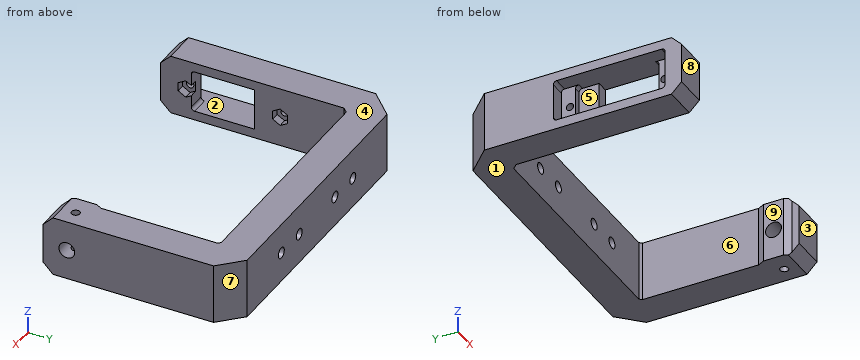
```python
from build123d import *

# Parameters (mm, degrees)
BOSS_EXTRUDE1_DEPTH             = 9
SKETCH2_R                       = 0.5
CUT_EXTRUDE1_DEPTH              = 67.414213562
SKETCH9_R                       = 2.38125
PIN_HOLE_DEPTH                  = 93.121320344
SKETCH20_R                      = 1.21925
SPRING_PIN_DEPTH                = 10
SPRING_PIN_DEPTH_BACK           = 10
SKETCH32_W                      = 12.5
SKETCH32_H                      = 33.5
CUT_EXTRUDE11_DEPTH             = 4.5
CUT_EXTRUDE12_REACH             = 89.621
SKETCH33_W                      = 12.5
SKETCH33_H                      = 25
CUT_EXTRUDE13_REACH             = 89.621
SKETCH34_R                      = 1.1
FILLET1_R                       = 1
TAP_DRILL_FOR_M4X0_7_TAP1_D     = 3.3
TAP_DRILL_FOR_M4X0_7_TAP1_DEPTH = 66.414213562
SKETCH41_W                      = 12.5
SKETCH41_H                      = 6
BOSS_EXTRUDE4_DEPTH             = 3.5
CUT_EXTRUDE14_DEPTH             = 2.5
BOSS_EXTRUDE6_DEPTH             = 9
CHAMFER1_SIZE                   = 3
CUT_EXTRUDE15_REACH             = 84.121
SKETCH45_R                      = 2.38125


with BuildPart() as part:
    # Sketch1 → Boss-Extrude1 (new body, symmetric)
    with BuildSketch(Plane.XY):
        Polygon((-35, 0), (35, 0), (35.707106781, -0.707106781), (35.707106781, -47.707106781), (45.707106781, -47.707106781), (45.707106781, 3.435028843), (39.142135624, 10), (-39.142135624, 10), (-46.414213562, 2.727922061), (-46.414213562, -56.414213562), (-36.414213562, -56.414213562), (-36.414213562, -1.414213562), align=None)
    extrude(amount=BOSS_EXTRUDE1_DEPTH, both=True)

    # Sketch2 → Cut-Extrude1 (cut, through all)
    with BuildSketch(Plane(origin=(0, 10, 0), x_dir=(1, 0, 0), z_dir=(0, 1, 0))):
        with Locations((-10, 0)):
            Circle(SKETCH2_R)
        with Locations((10, 0)):
            Circle(SKETCH2_R)
        with Locations((-20, 0)):
            Circle(SKETCH2_R)
        with Locations((20, 0)):
            Circle(SKETCH2_R)
    extrude(amount=-CUT_EXTRUDE1_DEPTH, mode=Mode.SUBTRACT)

    # Sketch9 → Pin Hole (cut, through all)
    with BuildSketch(Plane(origin=(45.707106781, 0, 0), x_dir=(0, 0, -1), z_dir=(1, 0, 0))):
        with Locations((0, -40.564971157)):
            Circle(SKETCH9_R)
    extrude(amount=-PIN_HOLE_DEPTH, mode=Mode.SUBTRACT)

    # Sketch20 → spring pin (cut, two sides)
    with BuildSketch(Plane.XY) as spring_pin_sk:
        with Locations((40.707106781, -40.564971157)):
            Circle(SKETCH20_R)
    extrude(amount=SPRING_PIN_DEPTH, mode=Mode.SUBTRACT)
    extrude(spring_pin_sk.sketch, amount=-SPRING_PIN_DEPTH_BACK, mode=Mode.SUBTRACT)

    # Sketch32 → Cut-Extrude11 (cut)
    with BuildSketch(Plane.ZY.offset(46.414213562)):
        with Locations((0, -34.734971157)):
            Rectangle(SKETCH32_W, SKETCH32_H)
    extrude(amount=-CUT_EXTRUDE11_DEPTH, mode=Mode.SUBTRACT)

    # Sketch33 → Cut-Extrude12 (cut, up to next)
    with BuildSketch(Plane.ZY.offset(41.914213562), mode=Mode.PRIVATE) as cut_extrude12_sk1:
        with Locations((0, -34.734971157)):
            Rectangle(SKETCH33_W, SKETCH33_H)
    cut_extrude12_tool1 = extrude(cut_extrude12_sk1.sketch, amount=-CUT_EXTRUDE12_REACH, mode=Mode.PRIVATE) & part.part
    add(cut_extrude12_tool1.solids().sort_by_distance((-41.914214, -34.734971, 0))[0], mode=Mode.SUBTRACT)

    # Sketch34 → Cut-Extrude13 (cut, up to next)
    with BuildSketch(Plane.ZY.offset(41.914213562), mode=Mode.PRIVATE) as cut_extrude13_sk1:
        with Locations((0, -20.574371157)):
            Circle(SKETCH34_R)
    cut_extrude13_tool1 = extrude(cut_extrude13_sk1.sketch, amount=-CUT_EXTRUDE13_REACH, mode=Mode.PRIVATE) & part.part
    add(cut_extrude13_tool1.solids().sort_by_distance((-41.914214, -20.574371, 0))[0], mode=Mode.SUBTRACT)
    # Sketch34 → Cut-Extrude13 (cut, up to next)
    with BuildSketch(Plane.ZY.offset(41.914213562), mode=Mode.PRIVATE) as cut_extrude13_sk2:
        with Locations((0, -48.895371157)):
            Circle(SKETCH34_R)
    cut_extrude13_tool2 = extrude(cut_extrude13_sk2.sketch, amount=-CUT_EXTRUDE13_REACH, mode=Mode.PRIVATE) & part.part
    add(cut_extrude13_tool2.solids().sort_by_distance((-41.914214, -48.895371, 0))[0], mode=Mode.SUBTRACT)

    # Fillet1
    fillet1_edges = [part.edges().sort_by_distance(p)[0] for p in [
        (-44.164213562, -17.984971157, 6.25),
        (-44.164213562, -51.484971157, 6.25),
        (-44.164213562, -51.484971157, -6.25),
        (-44.164213562, -17.984971157, -6.25),
        (-39.164213562, -22.234971157, -6.25),
        (-39.164213562, -47.234971157, -6.25),
        (-39.164213562, -47.234971157, 6.25),
        (-39.164213562, -22.234971157, 6.25),
    ]]
    fillet(fillet1_edges, radius=FILLET1_R)

    # Tap Drill for M4x0.7 Tap1
    with Locations(Plane(origin=(0, 10, 0), x_dir=(1, 0, 0), z_dir=(0, 1, 0))):
        with Locations((-20, 0), (20, 0), (-10, 0), (10, 0)):
            Hole(TAP_DRILL_FOR_M4X0_7_TAP1_D / 2, depth=TAP_DRILL_FOR_M4X0_7_TAP1_DEPTH)

    # Sketch41 → Boss-Extrude4 (add)
    with BuildSketch(Plane(origin=(-36.414213562, 0, 0), x_dir=(0, 0, -1), z_dir=(1, 0, 0))):
        with Locations((0, -25.234971157)):
            Rectangle(SKETCH41_W, SKETCH41_H)
    extrude(amount=-BOSS_EXTRUDE4_DEPTH)

    # Sketch43 → Cut-Extrude14 (cut)
    with BuildSketch(Plane(origin=(-36.414213562, 0, 0), x_dir=(0, 0, -1), z_dir=(1, 0, 0))):
        Polygon((-1.299038106, -22.824371157), (1.299038106, -22.824371157), (2.598076211, -20.574371157), (1.299038106, -18.324371157), (-1.299038106, -18.324371157), (-2.598076211, -20.574371157), align=None)
        Polygon((-1.299038106, -46.645371157), (-2.598076211, -48.895371157), (-1.299038106, -51.145371157), (1.299038106, -51.145371157), (2.598076211, -48.895371157), (1.299038106, -46.645371157), align=None)
    extrude(amount=-CUT_EXTRUDE14_DEPTH, mode=Mode.SUBTRACT)

    # Sketch44 → Boss-Extrude6 (add, symmetric)
    with BuildSketch(Plane.XY):
        Polygon((34.707106781, -37.564971157), (34.707106781, -40.564971157), (35.707106781, -40.564971157), (35.707106781, -35.564971157), align=None)
        Polygon((34.707106781, -40.564971157), (34.707106781, -43.564971157), (35.707106781, -45.564971157), (35.707106781, -40.564971157), align=None)
    extrude(amount=BOSS_EXTRUDE6_DEPTH, both=True)

    # Chamfer1
    chamfer1_edges = [part.edges().sort_by_distance(p)[0] for p in [
        (40.707106781, -47.707106781, -9),
        (40.707106781, -47.707106781, 9),
        (-41.414213562, -56.414213562, -9),
        (-41.414213562, -56.414213562, 9),
    ]]
    chamfer(chamfer1_edges, length=CHAMFER1_SIZE)

    # Sketch45 → Cut-Extrude15 (cut, up to next)
    with BuildSketch(Plane(origin=(35.707106781, 0, 0), x_dir=(0, 0, -1), z_dir=(1, 0, 0)), mode=Mode.PRIVATE) as cut_extrude15_sk1:
        with Locations((0, -40.564971157)):
            Circle(SKETCH45_R)
    cut_extrude15_tool1 = extrude(cut_extrude15_sk1.sketch, amount=-CUT_EXTRUDE15_REACH, mode=Mode.PRIVATE) & part.part
    add(cut_extrude15_tool1.solids().sort_by_distance((35.707107, -40.564971, 0))[0], mode=Mode.SUBTRACT)


solid = part.part
```
Model file for the job. Use its own axes, mm. Face numbers are marked on the shaded views. A direction names the side the tool comes from. Round coordinates to 2 decimals unless told otherwise and drop trailing zeros. Write each loop counter-clockwise with the first axis right and the second up, starting at its lowest first coordinate (ties: lowest second). Pieces come first, ordered by that corner, then holes. Notation, with made-up numbers: (56.25, 69) - (81.25, 69) arc R19 ccw to (81.25, 102) - close; hole circle Ø4 at (84, -16.75). An arc over 180 degrees is marked (long way). One line per item, written item: value.
(1) 3-axis set-ups, long thin cutter, end or side, ignore diameter. For the marked faces 5, 6, 7, 8 and 9: which of +Z, -Z, +X, -X, +Y, -Y reach the whole face in a straight line?
Values follow:
face 5: -X
face 6: +Z, -Z
face 7: +Z, -Z, +X, +Y
face 8: +Z, -Z, +X, -X, -Y
face 9: +Z, -Z, -Y
(2) Two-plate mould, pull along Z, no slides. Class the marked faces 1, 2, 3 and 4: pulls with the +Z half, pulls with the -Z half, needs draft (parallel to the pull), parting line crosses it, or undercut.
Values follow:
face 1: pulls with the -Z half
face 2: undercut
face 3: needs draft
face 4: pulls with the +Z half
(3) Cut at A-A, the plane y = -32.5. Give the cut face in (x, z), plus the area to 3 significant figures.
Values follow:
outline: (-46.41, -9) - (-36.41, -9) - (-36.41, -6.25) - (-46.41, -6.25) - close; (-46.41, 6.25) - (-36.41, 6.25) - (-36.41, 9) - (-46.41, 9) - close; (35.71, -9) - (45.71, -9) - (45.71, 9) - (35.71, 9) - close
area: 235 mm²
(4) Cut at B-B, the plane x = -10. Give the cut face in (y, z), plus the area to 3 significant figures.
Values follow:
outline: (0, -9) - (10, -9) - (10, -1.65) - (0, -1.65) - close; (0, 1.65) - (10, 1.65) - (10, 9) - (0, 9) - close
area: 147 mm²
(5) Drop flat-ended pins along their axis: P1, Ø1.8, axis at y = -40, z = 3.5, coming from the -X side; P2, Ø2.5, axis at y = -21.5, z = 0, coming from the -X side; P3, Ø3, axis at x = 10, z = 0, coming from the +Y side; P4, Ø5, axis at x = -44, z = 1.5, coming from the +Y side. Give the stop position or say it passes through.
Values follow:
P1: stops at x = 34.71
P2: stops at x = -41.91
P3: passes through
P4: stops at y = 7.64
(6) Wall check: probe 1 along Z at (x, y) = (10, 5); probe 2 along X at (y, z) = (-13, 2.5); probe 3 along X at (y, z) = (-25, -1.5). Give the ranges that are in metal, low to high.
Values follow:
probe 1: z = -9 to -1.65, 1.65 to 9
probe 2: x = -46.41 to -36.41, 35.71 to 45.71
probe 3: x = -39.91 to -36.41, 35.71 to 45.71
(7) Cut at C-C, the plane z = 0. Give the number of separate pieces and of enclosed holes in the cut face, plus the area to 3 significant figures.
Values follow:
separate pieces: 9
enclosed holes: 0
area: 1,440 mm²
